The listing builds one solid part. Answer for the finished solid, in the listing's coordinates (mm). Face numbers are marked on the shaded views. Coordinates: 2 decimals unless noted, no trailing zeros. Order: outer loops, then holes, each group sorted by start corner. A loop starts at its lowest first (then second) coordinate and runs counter-clockwise, first axis right, second up. Notation, with made-up numbers: M -20.5,44 L 36.5,44 A28 ccw 36.5,64 Z; hole C -7,-26 d8. An arc over 180 degrees is marked long. One line per item, written item: value. Start each with the question number.
Q1. The part is cut by section D-D on x = 2.5. Give the vertices of the cut face in (y, z), then the cut area to 3 significant figures.
Q2. The part is cut by section A-A on z = -31.5. Give the vertices of the cut face in (x, y).
Q3. Each of these flat-tipped pins is pushed along its axis until it touches: pin 1 Ø3 at (x, z) = (36, 46.5) entering from -Y; pin 2 Ø3 at (x, z) = (14, -39) entering from -Y; pin 3 Ø3.5 at (x, z) = (9.5, 64) entering from -Y; pin 4 Ø2 at (x, y) = (68.5, -9) entering from -Z. Where does it stop, or does it pass through?
Q4. Determine the mould class of the marked faces 1, 2 and 3 for opening direction Z: pulls with the +Z half, pulls with the -Z half, needs draft (parallel to the pull), parting line crosses it, or undercut.
Q5. The part is cut by section B-B on x = 63. Give the vertices of the cut face in (y, z).
Q6. The part is cut by section C-C on y = -2. Give the number of separate pieces and of enclosed holes in the cut face, then the cut area to 3 significant figures.
Q7. Straight lines are drawn through the part: line 1 along X through (y, z) = (-4.5, 0); line 2 along X through (y, z) = (-2.5, 24); line 3 along X through (y, z) = (-3, -16). For each, find the intervals that lie inside material, in ascending order. Write a range as [from, to].
```python
from build123d import *

# Parameters (mm, degrees)
F1_DEPTH = 99.25
F4_DEPTH = 2
F6_DEPTH = 12
F8_DEPTH = 10


# Not quite as in the source:
# - a feature names something its author has since deleted; it is built from what else it names


with BuildPart() as f1:
    # F0 (on Right) → F1 (new body, symmetric)
    with BuildSketch(Plane.YZ):
        with BuildLine():
            Line((0, 0), (0, 66))
            Line((0, 66), (-18, 71.8485545322))
            Line((-18, 71.8485545322), (-18, 61))
            Line((-18, 61), (-10, 61))
            ThreePointArc((-10, 61), (-6.4644660941, 59.5355339059), (-5, 56))
            Line((-5, 56), (-5, 0))
            Line((-5, 0), (0, 0))
        make_face()
        with BuildLine():
            Line((0, -66), (0, 0))
            Line((0, 0), (-5, 0))
            Line((-5, 0), (-5, -56))
            ThreePointArc((-5, -56), (-6.4644660941, -59.5355339059), (-10, -61))
            Line((-10, -61), (-18, -61))
            Line((-18, -61), (-18, -71.8485545322))
            Line((-18, -71.8485545322), (0, -66))
        make_face()
    extrude(amount=F1_DEPTH, both=True)

    # F3 (on face) + F2 (on face) → F4 (join)
    with BuildSketch(Plane.XZ.offset(18)):
        with BuildLine():
            ThreePointArc((-76.75, -66.4242772661), (-77.482233047, -64.6565103131), (-79.25, -63.9242772661))
            Line((-79.25, -63.9242772661), (-79.25, -68.9242772661))
            ThreePointArc((-79.25, -68.9242772661), (-77.482233047, -68.1920442191), (-76.75, -66.4242772661))
        make_face()
        with BuildLine():
            Line((-79.25, -68.9242772661), (-79.25, -63.9242772661))
            ThreePointArc((-79.25, -63.9242772661), (-81.75, -66.4242772661), (-79.25, -68.9242772661))
        make_face()
        with BuildLine():
            ThreePointArc((81.75, -66.4242772661), (81.017766953, -64.6565103131), (79.25, -63.9242772661))
            Line((79.25, -63.9242772661), (79.25, -68.9242772661))
            ThreePointArc((79.25, -68.9242772661), (81.017766953, -68.1920442191), (81.75, -66.4242772661))
        make_face()
        with BuildLine():
            Line((79.25, -68.9242772661), (79.25, -63.9242772661))
            ThreePointArc((79.25, -63.9242772661), (76.75, -66.4242772661), (79.25, -68.9242772661))
        make_face()
    with BuildSketch(Plane.XZ.offset(18)):
        with BuildLine():
            Line((-79.25, 63.9242772661), (-79.25, 68.9242772661))
            ThreePointArc((-79.25, 68.9242772661), (-81.75, 66.4242772661), (-79.25, 63.9242772661))
        make_face()
        with BuildLine():
            ThreePointArc((-76.75, 66.4242772661), (-77.482233047, 68.1920442191), (-79.25, 68.9242772661))
            Line((-79.25, 68.9242772661), (-79.25, 63.9242772661))
            ThreePointArc((-79.25, 63.9242772661), (-77.482233047, 64.6565103131), (-76.75, 66.4242772661))
        make_face()
        with BuildLine():
            Line((79.25, 63.9242772661), (79.25, 68.9242772661))
            ThreePointArc((79.25, 68.9242772661), (76.75, 66.4242772661), (79.25, 63.9242772661))
        make_face()
        with BuildLine():
            ThreePointArc((81.75, 66.4242772661), (81.017766953, 68.1920442191), (79.25, 68.9242772661))
            Line((79.25, 68.9242772661), (79.25, 63.9242772661))
            ThreePointArc((79.25, 63.9242772661), (81.017766953, 64.6565103131), (81.75, 66.4242772661))
        make_face()
    extrude(amount=F4_DEPTH)

    # F5 (on face) → F6 (cut)
    with BuildSketch(Plane(origin=(0, 19.3969133257, 59.6975608144), x_dir=(1, 0, 0), z_dir=(0, 0.3090169944, 0.9510565163))):
        with BuildLine():
            Line((-31.25, -26.321441665), (-71.25, -26.321441665))
            ThreePointArc((-71.25, -26.321441665), (-74.7855339059, -27.7859077591), (-76.25, -31.321441665))
            Line((-76.25, -31.321441665), (-76.25, -39.321441665))
            Line((-76.25, -39.321441665), (-26.25, -39.321441665))
            Line((-26.25, -39.321441665), (-26.25, -31.321441665))
            ThreePointArc((-26.25, -31.321441665), (-27.7144660941, -27.7859077591), (-31.25, -26.321441665))
        make_face()
    extrude(amount=-F6_DEPTH, mode=Mode.SUBTRACT)

    # F7 (on face) → F8 (cut)
    with BuildSketch(Plane(origin=(0, 0, 0), x_dir=(-1, 0, 0), z_dir=(0, 1, 0))):
        with BuildLine():
            Line((-26.1241253117, 43.5324917753), (-39.945202857, 41.7259457748))
            ThreePointArc((-39.945202857, 41.7259457748), (-42.868486138, 40.2675021288), (-44.2671531873, 37.3151516253))
            Line((-44.2671531873, 37.3151516253), (-51.2410791047, -26.0453891719))
            ThreePointArc((-51.2410791047, -26.0453891719), (-47.4179750613, -37.7900376772), (-36.0778427088, -42.6843498113))
            Line((-36.0778427088, -42.6843498113), (4.1248849593, -42.0054160058))
            ThreePointArc((4.1248849593, -42.0054160058), (5.4117305762, -41.5076906746), (6.0700611664, -40.2951301685))
            Line((6.0700611664, -40.2951301685), (7.9760571648, -27.2630410602))
            ThreePointArc((7.9760571648, -27.2630410602), (7.4832995732, -25.6352393882), (5.915823381, -24.9752646049))
            Line((5.915823381, -24.9752646049), (-24.1576078612, -26.198563135))
            ThreePointArc((-24.1576078612, -26.198563135), (-29.5966863815, -23.9404174945), (-31.3872943296, -18.3300235635))
            Line((-31.3872943296, -18.3300235635), (-23.8805734625, 41.2995541596))
            ThreePointArc((-23.8805734625, 41.2995541596), (-24.45405494, 42.9669237235), (-26.1241253117, 43.5324917753))
        make_face()
        with BuildLine():
            ThreePointArc((-5.7212161103, 40.5873727881), (-6.9681438523, 40.0278262586), (-7.5645672745, 38.7981107574))
            Line((-7.5645672745, 38.7981107574), (-12.0217983934, -4.3736584849))
            ThreePointArc((-12.0217983934, -4.3736584849), (-10.3919235454, -9.1345167822), (-5.7104341995, -10.9800305997))
            Line((-5.7104341995, -10.9800305997), (26.823213324, -9.1166598722))
            Line((26.823213324, -9.1166598722), (23.9718645269, -39.7895195484))
            ThreePointArc((23.9718645269, -39.7895195484), (24.4850628135, -41.3218155235), (25.9632785739, -41.9746413827))
            Line((25.9632785739, -41.9746413827), (39.8267463101, -41.9746413827))
            ThreePointArc((39.8267463101, -41.9746413827), (41.1595537584, -41.4658235666), (41.8142050316, -40.1982656883))
            Line((41.8142050316, -40.1982656883), (50.9657841779, 41.1363000735))
            ThreePointArc((50.9657841779, 41.1363000735), (50.3629399127, 42.8031301188), (48.6725697432, 43.3364145622))
            Line((48.6725697432, 43.3364145622), (33.3066192392, 40.9593589134))
            ThreePointArc((33.3066192392, 40.9593589134), (32.1599535015, 40.357813067), (31.6221064236, 39.1799250248))
            Line((31.6221064236, 39.1799250248), (28.5455137491, 8.1063397229))
            Line((28.5455137491, 8.1063397229), (8.093200624, 7.1375463158))
            Line((8.093200624, 7.1375463158), (12.000094254, 39.4946401574))
            ThreePointArc((12.000094254, 39.4946401574), (11.4616105973, 41.1149341717), (9.8684416836, 41.7290434075))
            Line((9.8684416836, 41.7290434075), (-5.7212161103, 40.5873727881))
        make_face()
    extrude(amount=-F8_DEPTH, mode=Mode.SUBTRACT)


solid = f1.part
```
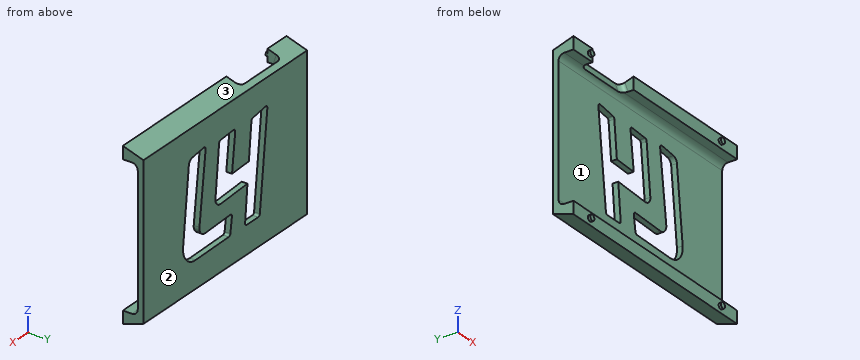
Output:
1. outline: M -18,-71.85 L 0,-66 L 0,-42.12 L -5,-42.12 L -5,-56 A5 cw -10,-61 L -18,-61 Z; M -18,61 L -10,61 A5 cw -5,56 L -5,40.82 L 0,40.82 L 0,66 L -18,71.85 Z; M -5,-25.32 L 0,-25.32 L 0,-10.8 L -5,-10.8 Z
1. area: 564 mm^2
2. outline: M -99.25,-5 L -42.79,-5 L -42.79,0 L -99.25,0 Z; M -24.74,-5 L -7.36,-5 L -7.36,0 L -24.74,0 Z; M 50.84,-5 L 99.25,-5 L 99.25,0 L 50.84,0 Z
3. pin 1: stops at y = -5
3. pin 2: passes through
3. pin 3: stops at y = -18
3. pin 4: stops at z = -69.25
4. face 1: undercut
4. face 2: needs draft
4. face 3: pulls with the +Z half
5. outline: M -18,-71.85 L 0,-66 L 0,66 L -18,71.85 L -18,61 L -10,61 A5 cw -5,56 L -5,-56 A5 cw -10,-61 L -18,-61 Z
6. separate pieces: 1
6. enclosed holes: 2
6. area: 21,300 mm^2
7. line 1: x = [-99.25, -46.34], [11.57, 29.08], [48.37, 99.25]
7. line 2: x = [-99.25, -49.04], [-30.12, -10.13], [9.09, 26.06], [45.73, 99.25]
7. line 3: x = [-99.25, -44.54], [-26.18, 31.09], [50.14, 99.25]
